Read the model definition and answer for the solid it produces. Units are mm, in the model's axes. A direction names the side the tool comes from. Give positions to 0.01 mm unless a question says otherwise; leave off trailing zeros. Order: outer loops, then holes, each group sorted by start corner. A loop starts at its lowest first (then second) coordinate and runs counter-clockwise, first axis right, second up. Notation, with made-up numbers: M 7,-38.75 L 14,-38.75 A15 cw 14,-32.75 Z; hole C 64.5,49 d5. An arc over 180 degrees is marked long. Write item = value, one per line. Start each with the question number.
Autodesk Inventor part; units mm, degrees
ref_plane "YZ Plane" through (0, 0, 0) normal (1, 0, 0) x (0, 1, 0)
ref_plane "XZ Plane" through (0, 0, 0) normal (0, 1, 0) x (-1, 0, 0)
ref_plane "XY Plane" through (0, 0, 0) normal (0, 0, 1) x (1, 0, 0)
sketch "Szkic1" plane through (0, 0, 0) normal (0, 0, 1) x (1, 0, 0)
  line L0 (0, 0) -> (34, 0)
  line L1 (34, 0) -> (34, 10)
  line L2 (34, 10) -> (0, 10)
  line L3 (0, 10) -> (0, 0)
  circle A0 centre (34, 10) radius 10
  point P0 (24, 10)
  dimension "d0" = 34
  dimension "d1" = 10
  dimension "d2" = 20
extrude "Wyciągnięcie proste1" add sketch "Szkic1" along normal mid plane 26
chamfer "Faza1" distance 4 angle 45 1 edges at (0, 0, 0)
sketch "Szkic2" plane through (0, 0, 13) normal (0, 0, 1) x (1, 0, 0)
  arc A0 (34, 0) -> (24, 10) centre (34, 10) ccw
  point P0 (0, 0)
hole "Otwór1" at (34, 10, 13) direction (0, 0, -1) diameter 12.5 end through all
sketch "Szkic3" plane through (0, 10, 13) normal (0, 1, 0) x (1, 0, 0)
  line L0 (0, 18) -> (12, 18)
  line L1 (12, 18) -> (12, 8)
  line L2 (12, 8) -> (0, 8)
  line L3 (0, 8) -> (0, 18)
  circle A0 centre (12, 13) radius 5
  point P0 (0, 13)
extrude "Wyciągnięcie proste2" cut sketch "Szkic3" against normal through all
1) Each of these flat-tipped pins is pushed along its axis until it touches: P1, Ø2, axis at x = 17, z = -7, coming from the -Y side; P2, Ø1.5, axis at x = 24, y = 15.5, coming from the -Z side. Where does it stop, or does it pass through?
2) Find the intervals of material crossed by probe 1 along Y at (x, z) = (34, 5.75); probe 2 along Z at (x, y) = (8.5, 2.25); probe 3 along X at (y, z) = (15.5, 4.25), in increasing order. Write a range as [from, to].
3) For a pull along Z with two mould halves and no side action, classify faces 4 (the face through (6, 5, -5)), 5 (the face through (22, 8, 13)), 6 (the face through (2, 2, 9)) as pulls with the +Z half, pulls with the -Z half, needs draft (parallel to the pull), parting line crosses it, or undercut.
4) Find section C-C on z = -7.25. Determine the outline of the cut face in (x, y), plus the area to 3 significant figures.
5) Find section D-D on y = 1.5. Determine the outline of the cut face in (x, z).
6) Find section B-B on y = 7. Determine the outline of the cut face in (x, z).
7) For faces 1 (the face through (18, 10, 0)), 2 (the face through (0, 7, 9)), 3 (the face through (6, 5, 5)), determine the directions among +Z, -Z, +X, -X, +Y, -Y from which every point of the face is accessible in a straight line to the end or side of a thin tool.
8) Find section A-A on x = 39. Determine the outline of the cut face in (y, z).
Numbers:
q1.P1 = 0
q1.P2 = through
q2.probe_1 = [0, 3.75], [16.25, 20]
q2.probe_2 = [-13, -5], [5, 13]
q2.probe_3 = [25.65, 31.03], [36.97, 42.35]
q3.face_4 = undercut
q3.face_5 = pulls with the +Z half
q3.face_6 = needs draft
q4.outline = M 0,4 L 4,0 L 34,0 A10 ccw long 24,10 L 0,10 Z; hole C 34,10 d12.5
q4.area = 445 mm2
q5.outline = M 2.5,-13 L 39.27,-13 L 39.27,13 L 2.5,13 L 2.5,5 L 12,5 A5 cw 12,-5 L 2.5,-5 Z
q6.outline = M 0,-13 L 28.52,-13 L 28.52,13 L 0,13 L 0,5 L 12,5 A5 cw 12,-5 L 0,-5 Z; M 39.48,-13 L 43.54,-13 L 43.54,13 L 39.48,13 Z
q7.face_1 = +Z, -Z, -X, +Y
q7.face_2 = +Z, -Z, -X, +Y, -Y
q7.face_3 = -X, +Y, -Y
q8.outline = M 1.34,-13 L 6.25,-13 L 6.25,13 L 1.34,13 Z; M 13.75,-13 L 18.66,-13 L 18.66,13 L 13.75,13 Z
